from build123d import *

# Parameters (mm, degrees)
BOSS_EXTRUDE1_DEPTH = 5
BOSS_EXTRUDE2_DEPTH = 73
CUT_EXTRUDE1_DEPTH  = 68
BOSS_EXTRUDE3_DEPTH = 73
CUT_EXTRUDE3_DEPTH  = 73
CHAMFER1_SIZE       = 10


with BuildPart() as part:
    # Sketch3 → Boss-Extrude1 (new body)
    with BuildSketch(Plane(origin=(0, 0, 0), x_dir=(1, 0, 0), z_dir=(0, 1, 0))):
        Polygon((50.577269222, -29.2008), (50.577269222, 29.2008), (0, 58.4016), (-50.577269222, 29.2008), (-50.577269222, -29.2008), (0, -58.4016), align=None)
        Polygon((43.577269222, -25.159348116), (43.577269222, 25.159348116), (0, 50.318696231), (-43.577269222, 25.159348116), (-43.577269222, -25.159348116), (0, -50.318696231), align=None, mode=Mode.SUBTRACT)
    extrude(amount=BOSS_EXTRUDE1_DEPTH)

    # Sketch4 → Boss-Extrude2 (add)
    with BuildSketch(Plane(origin=(0, 5, 0), x_dir=(1, 0, 0), z_dir=(0, 1, 0))):
        Polygon((47.077269222, -27.180074058), (47.077269222, 27.180074058), (0, 54.360148116), (-47.077269222, 27.180074058), (-47.077269222, -27.180074058), (0, -54.360148116), align=None)
    extrude(amount=-BOSS_EXTRUDE2_DEPTH)

    # Sketch5 → Cut-Extrude1 (cut)
    with BuildSketch(Plane(origin=(0, 5, 0), x_dir=(1, 0, 0), z_dir=(0, 1, 0))):
        Polygon((43.577269222, -25.159348116), (43.577269222, 25.159348116), (0, 50.318696231), (-43.577269222, 25.159348116), (-43.577269222, -25.159348116), (0, -50.318696231), align=None)
    extrude(amount=-CUT_EXTRUDE1_DEPTH, mode=Mode.SUBTRACT)

    # Sketch6 → Boss-Extrude3 (add)
    with BuildSketch(Plane(origin=(0, 5, 0), x_dir=(1, 0, 0), z_dir=(0, 1, 0))):
        with BuildLine():
            ThreePointArc((-28.017982948, -34.142506234), (-29.520182072, -17.058341723), (-43.577269222, -7.233700248))
            Line((-43.577269222, -7.233700248), (-43.577269222, -25.159348116))
            Line((-43.577269222, -25.159348116), (-28.017982948, -34.142506234))
        make_face()
    extrude(amount=-BOSS_EXTRUDE3_DEPTH)

    # Sketch9 → Cut-Extrude3 (cut)
    with BuildSketch(Plane(origin=(0, 5, 0), x_dir=(1, 0, 0), z_dir=(0, 1, 0))):
        with BuildLine():
            Line((-47.077269222, -10.180074058), (-47.077269222, -27.180074058))
            Line((-47.077269222, -27.180074058), (-32.354837357, -35.680074058))
            ThreePointArc((-32.354837357, -35.680074058), (-32.354837357, -18.680074058), (-47.077269222, -10.180074058))
        make_face()
    extrude(amount=-CUT_EXTRUDE3_DEPTH, mode=Mode.SUBTRACT)

    # Chamfer1
    chamfer1_edges = [part.edges().sort_by_distance(p)[0] for p in [
        (21.788634611, -63, 37.739022174),
        (-43.577269222, -63, -8.962823934),
        (-21.788634611, -63, -37.739022174),
        (21.788634611, -63, -37.739022174),
        (43.577269222, -63, 0),
        (-14.008991474, -63, 42.230601233),
    ]]
    chamfer(chamfer1_edges, length=CHAMFER1_SIZE)


solid = part.part
The model under review builds one solid part; all positions refer to its coordinate system, in mm. A direction names the side the tool comes from. Give positions to 0.01 mm unless a question says otherwise; leave off trailing zeros. Write each loop counter-clockwise with the first axis right and the second up, starting at its lowest first coordinate (ties: lowest second). Pieces come first, ordered by that corner, then holes.
1. Draft analysis for pull direction X (two halves, no side actions). For faces 6 (the flat face through (-24.93, 2.46, -44.01)), 7 (the flat face through (23.21, -33.52, 40.96)), 8 (the flat face through (-13.87, -57.93, 36.62)), state which applies: +X half, -X half, draft (parallel to the pull), parting line (faces both ways), or undercut.
2. Add section D-D, the plane z = -22. Write out the cut boundary in (x, y).
3. For P1, Ø18.5, axis at y = -23, z = -0.5, coming from the -X side; P2, Ø10, axis at y = -30, z = -32.5, coming from the +X side; P3, Ø2, axis at y = -53.5, z = -37, coming from the +X side; P4, Ø8, axis at x = 8, z = 43.5, coming from the +Y side, all flat-tipped, find the tip position at first contact; note any pin that passes through.
4. Add section A-A, the plane y = -23. Write out the cut boundary in (x, z), plus the area to 3 significant figures.
5. Add section C-C, the plane x = -19.5. Write out the cut boundary in (y, z).
6. Tool access review of faces 1 (the flat face through (43.577, -24, 0)), 2 (the flat face through (-16.4, -33.52, 44.89)), 3 (the flat face through (-23, 0, 43)), 4 (the flat face through (-47.077, 3, 19)), 5 (the flat face through (23.87, -33.52, -40.58)): name each direction out of +Z, -Z, +X, -X, +Y, -Y from which nothing blocks a thin tool from reaching the whole face with its end or side.
7. Add section B-B, the plane z = -4. Write out the cut boundary in (x, y).
8. Wall thickness on L1, parallel to Y at x = 2.5, z = -9; L2, parallel to X at y = -6, z = 17.5; L3, parallel to Z at x = -35.5, y = -13: over which ranges is each line inside the solid? List them lowest first.
Worked answers:
1. face 6: -X half
1. face 7: +X half
1. face 8: undercut
2. outline: (-50.58, 0) - (-47.08, 0) - (-47.08, -68) - (47.08, -68) - (47.08, 0) - (50.58, 0) - (50.58, 5) - (43.58, 5) - (43.58, -53) - (38.11, -58.47) - (29.05, -63) - (-29.05, -63) - (-38.11, -58.47) - (-43.58, -53) - (-43.58, 5) - (-50.58, 5) - close
3. P1: stops at x = -47.08
3. P2: stops at x = 46.52
3. P3: stops at x = 31.8
3. P4: stops at y = 5
4. outline: (-47.08, -27.18) - (0, -54.36) - (47.08, -27.18) - (47.08, 27.18) - (0, 54.36) - (-32.35, 35.68) arc R17 cw to (-47.08, 10.18) - close; hole (-43.58, -25.16) - (0, -50.32) - (43.58, -25.16) - (43.58, 25.16) - (0, 50.32) - (-28.02, 34.14) arc R20.28 cw to (-43.58, 7.23) - close
4. area: 1,090 mm2
5. outline: (-68, -43.1) - (0, -43.1) - (0, -47.14) - (5, -47.14) - (5, -39.06) - (-53, -39.06) - (-63, -27.51) - (-63, 27.51) - (-53, 39.06) - (5, 39.06) - (5, 47.14) - (0, 47.14) - (0, 43.1) - (-68, 43.1) - close
6. face 1: +Y
6. face 2: +Z, -X, -Y
6. face 3: -Y
6. face 4: +Y, -Y
6. face 5: -Z, +X, -Y
7. outline: (-50.58, 0) - (-47.08, 0) - (-47.08, -68) - (47.08, -68) - (47.08, 0) - (50.58, 0) - (50.58, 5) - (43.58, 5) - (43.58, -53) - (33.58, -63) - (-33.58, -63) - (-43.58, -53) - (-43.58, 5) - (-50.58, 5) - close
8. L1: y = -68 to -63
8. L2: x = -33.1 to -29.27, 43.58 to 47.08
8. L3: z = -33.86 to -29.82, 10.56 to 14.73
